Build history of the part. All positions in model axes, mm. A direction names the side the tool comes from. Round coordinates to 2 decimals unless told otherwise and drop trailing zeros. Loops run counter-clockwise (first coordinate to the right, second up) from the corner with the lowest first, then second, coordinate; pieces in that order, holes last.
from build123d import *

# Parameters (mm, degrees)
F1_DEPTH = 50.8
F2_R     = 6.35
F3_DEPTH = 101.601


with BuildPart() as f1:
    # F0 (on Front) → F1 (new body, symmetric)
    with BuildSketch(Plane.XZ):
        Polygon((38.1, 47.625), (38.1, 50.8), (-38.1, 50.8), (-38.1, -50.8), (38.1, -50.8), (38.1, -47.625), (-34.925, -47.625), (-34.925, 47.625), align=None)
    extrude(amount=F1_DEPTH, both=True)

    # F2 (on face) → F3 (cut, through all)
    with BuildSketch(Plane(origin=(0, 0, -50.8), x_dir=(1, 0, 0), z_dir=(0, 0, -1))):
        Circle(F2_R)
    extrude(amount=-F3_DEPTH, mode=Mode.SUBTRACT)


solid = f1.part
(1) Slice it at B-B on x = 0. List the corners of the cut face in (y, z) (3 decimals).
Responses:
outline: (-50.8, -50.8) - (-6.35, -50.8) - (-6.35, -47.625) - (-50.8, -47.625) - close; (-50.8, 47.625) - (-6.35, 47.625) - (-6.35, 50.8) - (-50.8, 50.8) - close; (6.35, -50.8) - (50.8, -50.8) - (50.8, -47.625) - (6.35, -47.625) - close; (6.35, 47.625) - (50.8, 47.625) - (50.8, 50.8) - (6.35, 50.8) - close
(2) Slice it at C-C on x = 33. List the corners of the cut face in (y, z) (3 decimals).
Responses:
outline: (-50.8, -50.8) - (50.8, -50.8) - (50.8, -47.625) - (-50.8, -47.625) - close; (-50.8, 47.625) - (50.8, 47.625) - (50.8, 50.8) - (-50.8, 50.8) - close
(3) Pull direction Y, two halves, no side cores. Call faces 3 (the face through (-37, 50.8, 0)), 4 (the face through (38.1, -1, -49)), 5 (the face through (-1.38, 6.2, -49.23)): +Y half, -Y half, draft (parallel to the pull), parting line (faces both ways), or undercut.
Responses:
face 3: +Y half
face 4: draft
face 5: undercut
(4) Probe line 1 (Z direction, x = 1, y = -23.5) (3 decimals); line 2 (X direction, y = 0, z = -48.5); line 3 (Y direction, x = 0, z = 49.9). List the from-to ranges inside material, lowest first.
Responses:
line 1: z = -50.8 to -47.625, 47.625 to 50.8
line 2: x = -38.1 to -6.35, 6.35 to 38.1
line 3: y = -50.8 to -6.35, 6.35 to 50.8
(5) Slice it at A-A on y = 0. List the corners of the cut face in (x, z) (3 decimals), plus the area to 3 significant figures.
Responses:
outline: (-38.1, -50.8) - (-6.35, -50.8) - (-6.35, -47.625) - (-34.925, -47.625) - (-34.925, 47.625) - (-6.35, 47.625) - (-6.35, 50.8) - (-38.1, 50.8) - close; (6.35, -50.8) - (38.1, -50.8) - (38.1, -47.625) - (6.35, -47.625) - close; (6.35, 47.625) - (38.1, 47.625) - (38.1, 50.8) - (6.35, 50.8) - close
area: 706 mm2
(6) Pin check, flat tip, straight feed: P1, Ø10, axis at x = 0, y = 0, coming from the -Z side. Stop position of the tip, or through.
Responses:
P1: passes through
(7) Slice it at D-D on y = 29. List the corners of the cut face in (x, z) (3 decimals).
Responses:
outline: (-38.1, -50.8) - (38.1, -50.8) - (38.1, -47.625) - (-34.925, -47.625) - (-34.925, 47.625) - (38.1, 47.625) - (38.1, 50.8) - (-38.1, 50.8) - close
(8) Which spindle directions (+Z, -Z, +X, -X, +Y, -Y) get a long thin tool onto all of the face, cutting with end or side? Do faces 1 (the face through (-8, -1, 50.8)), 2 (the face through (10, -1, -47.625)). Say none if no direction does.
Responses:
face 1: +Z, +X, -X, +Y, -Y
face 2: +X, +Y, -Y
